from build123d import *

# Parameters (mm, degrees)
SKETCH1_R           = 6
SKETCH1_W           = 65
SKETCH1_H           = 35
BOSS_EXTRUDE1_DEPTH = 20
SKETCH1_3_W         = 35
SKETCH1_3_H         = 35
SKETCH1_3_W_2       = 100
SKETCH1_3_H_2       = 20
BOSS_EXTRUDE2_DEPTH = 40
SKETCH3_W           = 10
SKETCH3_H           = 10
BOSS_EXTRUDE4_DEPTH = 100
CUT_EXTRUDE1_DEPTH  = 65


with BuildPart() as part:
    # Sketch1 → Boss-Extrude1 (new body)
    with BuildSketch(Plane.XY):
        Polygon((100, -20), (0, -20), (0, -45), (35, -45), (100, -45), align=None)
        with Locations((15, -32.5)):
            Circle(SKETCH1_R, mode=Mode.SUBTRACT)
        with Locations((75, -32.5)):
            Circle(SKETCH1_R, mode=Mode.SUBTRACT)
        with Locations((67.5, -62.5)):
            Rectangle(SKETCH1_W, SKETCH1_H)
    extrude(amount=BOSS_EXTRUDE1_DEPTH)

    # Sketch1<3> → Boss-Extrude2 (add)
    with BuildSketch(Plane.XY):
        with Locations((17.5, -62.5)):
            Rectangle(SKETCH1_3_W, SKETCH1_3_H)
        with Locations((50, -10)):
            Rectangle(SKETCH1_3_W_2, SKETCH1_3_H_2)
    extrude(amount=BOSS_EXTRUDE2_DEPTH)

    # Sketch3 → Boss-Extrude4 (add)
    with BuildSketch(Plane(origin=(0, 0, 0), x_dir=(0, 0, -1), z_dir=(1, 0, 0))):
        with Locations((5, -75)):
            Rectangle(SKETCH3_W, SKETCH3_H)
        with Locations((5, -5)):
            Rectangle(SKETCH3_W, SKETCH3_H)
    extrude(amount=BOSS_EXTRUDE4_DEPTH)

    # Sketch4 → Cut-Extrude1 (cut)
    with BuildSketch(Plane(origin=(100, 0, 0), x_dir=(0, 0, -1), z_dir=(1, 0, 0))):
        Polygon((-20, -45), (0, -80), (-20, -80), align=None)
    extrude(amount=-CUT_EXTRUDE1_DEPTH, mode=Mode.SUBTRACT)


solid = part.part
Can you work these out from the model? Positions are in its coordinate system, mm. A direction names the side the tool comes from. Coordinates: 2 decimals unless noted, no trailing zeros. Order: outer loops, then holes, each group sorted by start corner. A loop starts at its lowest first (then second) coordinate and runs counter-clockwise, first axis right, second up. Notation, with made-up numbers: M 40,65 L 91,65 A11 ccw 91,77 Z; hole C 58.5,-6.75 d5. An arc over 180 degrees is marked long. Write item = value, one per line.
(1) If we mould it in two halves opening along Y, with no side actions, what happens to faces 1 (the face through (67.955, -62.255, 10.14)), 2 (the face through (17, -45, 30)), 3 (the face through (49, -5, -10))? For each: pulls with the +Y half, pulls with the -Y half, needs draft (parallel to the pull), parting line crosses it, or undercut.
Results are:
face_1 = pulls with the -Y half
face_2 = undercut
face_3 = needs draft
(2) Suppose I cut it at B-B on x = 75. Please give me the cut outline in (y, z), plus the area to 3 significant figures.
Results are:
outline = M -80,-10 L -70,-10 L -70,0 L -38.5,0 L -38.5,20 L -45,20 L -80,0 Z; M -26.5,0 L -10,0 L -10,-10 L 0,-10 L 0,40 L -20,40 L -20,20 L -26.5,20 Z
area = 1,610 mm2
(3) Suppose I cut it at C-C on y = -32.5. Please give me the cut outline in (x, z), plus the area to 3 significant figures.
Results are:
outline = M 0,0 L 9,0 L 9,20 L 0,20 Z; M 21,0 L 69,0 L 69,20 L 21,20 Z; M 81,0 L 100,0 L 100,20 L 81,20 Z
area = 1,520 mm2
(4) For faces 4 (the face through (49, -10, -5)), 5 (the face through (49, -20, 30)), 6 (the face through (35, -62, 24)), which set-ups out of +Z, -Z, +X, -X, +Y, -Y let a thin tool reach every point of the face, with its end or its side?
Results are:
face_4 = -Z, +X, -X
face_5 = +Z, +X, -X
face_6 = +Z, +X, -Y
(5) I need wall thicknesses on line 1 along X through (y, z) = (-32, 11); line 2 along X through (y, z) = (-34, 4); line 3 along Z through (x, y) = (6.5, -43). Which ranges of each line are inside material? Lowest first, please. Write a range as [from, to].
Results are:
line_1 = [0, 9.02], [20.98, 69.02], [80.98, 100]
line_2 = [0, 9.19], [20.81, 69.19], [80.81, 100]
line_3 = [0, 20]
(6) For pin 1 Ø15.5 at (x, y) = (75, -32.5) entering from -Z; pin 2 Ø3 at (x, z) = (42, 9.5) entering from -Y; pin 3 Ø22 at (x, z) = (70, 31.5) entering from -Y, each with a flat end and sliding along its axis, tell me the tip position at first contact or that it passes through.
Results are:
pin_1 = 0
pin_2 = -66
pin_3 = -20
(7) Suppose I cut it at A-A on z = -5. Please give me the cut outline in (x, y), plus the area to 3 significant figures.
Results are:
outline = M 0,-80 L 100,-80 L 100,-70 L 0,-70 Z; M 0,-10 L 100,-10 L 100,0 L 0,0 Z
area = 2,000 mm2
(8) Suppose I cut it at D-D on z = 6. Please give me the cut outline in (x, y), plus the area to 3 significant figures.
Results are:
outline = M 0,-80 L 35,-80 L 35,-69.5 L 100,-69.5 L 100,0 L 0,0 Z; hole C 15,-32.5 d12; hole C 75,-32.5 d12
area = 7,090 mm2
